```python
from build123d import *

# Parameters (mm, degrees)
F0_W     = 180.975
F0_H     = 146.05
F1_DEPTH = 19.05


with BuildPart() as f1:
    # F0 (on Top) → F1 (new body)
    with BuildSketch(Plane.XY):
        Polygon((284.226, -280.9875), (284.226, 280.9875), (233.426, 280.9875), (233.426, 242.8875), (-233.426, 242.8875), (-233.426, 280.9875), (-284.226, 280.9875), (-284.226, -280.9875), align=None)
        Rectangle(F0_W, F0_H, mode=Mode.SUBTRACT)
    extrude(amount=F1_DEPTH)


solid = f1.part
```
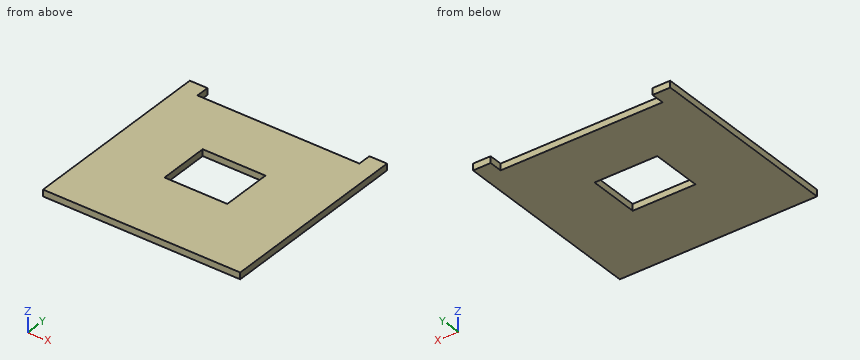
Work out the finished part from the listing and answer in its coordinate system (mm). Round coordinates to 2 decimals unless told otherwise and drop trailing zeros. Write each loop counter-clockwise with the first axis right and the second up, starting at its lowest first coordinate (ties: lowest second). Pieces come first, ordered by that corner, then holes.
1) Consider probe 1 along Y at (x, z) = (35, 5.75) (1 decimal); probe 2 along X at (y, z) = (-34.5, 17.5); probe 3 along Y at (x, z) = (-144.5, 10). Determine where each line is inside the solid, lowest interval first.
2) Flat-ended cylindrical pins translate along their axes: P1, Ø10, axis at x = 145.5, y = 129, coming from the -Z side; P2, Ø5, axis at x = 214.5, z = 16.5, coming from the +Y side. Find the tip coordinate at first contact, or state that the pin passes through.
3) A cutting plane is placed at D-D on x = 100.5. Determine the outline of the cut face in (y, z), and give its area (3 significant figures).
4) A cutting plane is placed at C-C on z = 16. Determine the outline of the cut face in (x, y) (1 decimal), and give its area (3 significant figures).
5) A cutting plane is placed at B-B on y = -20. Determine the outline of the cut face in (x, z).
Entries:
1. probe 1: y = -281 to -73, 73 to 242.9
1. probe 2: x = -284.23 to -90.49, 90.49 to 284.23
1. probe 3: y = -280.99 to 242.89
2. P1: stops at z = 0
2. P2: stops at y = 242.89
3. outline: (-280.99, 0) - (242.89, 0) - (242.89, 19.05) - (-280.99, 19.05) - close
3. area: 9,980 mm2
4. outline: (-284.2, -281) - (284.2, -281) - (284.2, 281) - (233.4, 281) - (233.4, 242.9) - (-233.4, 242.9) - (-233.4, 281) - (-284.2, 281) - close; hole (-90.5, -73) - (90.5, -73) - (90.5, 73) - (-90.5, 73) - close
4. area: 275,000 mm2
5. outline: (-284.23, 0) - (-90.49, 0) - (-90.49, 19.05) - (-284.23, 19.05) - close; (90.49, 0) - (284.23, 0) - (284.23, 19.05) - (90.49, 19.05) - close
